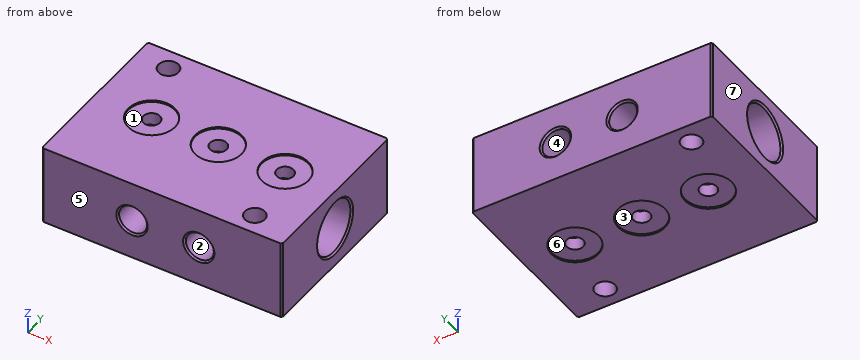
```python
from build123d import *

# Parameters (mm, degrees)
F0_W      = 35
F0_H      = 25
F1_DEPTH  = 12
F2_R      = 4
F3_DEPTH  = 35
F4_R      = 3.5
F4_R_2    = 1.25
F5_DEPTH  = 0.25
F4_R_3    = 1.5
F6_DEPTH  = 25
F7_R      = 1.25
F8_DEPTH  = 25
F10_R     = 2.1
F10_R_2   = 1.25
F11_DEPTH = 6
F9_R      = 2.1
F9_R_2    = 1.25
F12_DEPTH = 6
F13_DEPTH = 1
F14_SIZE  = 0.25
F15_SIZE  = 0.25


with BuildPart() as f1:
    # F0 (on Top) → F1 (new body)
    with BuildSketch(Plane.XY):
        with Locations((17.5, -12.5)):
            Rectangle(F0_W, F0_H)
    extrude(amount=F1_DEPTH)

    # F2 (on face) → F3 (cut, through all)
    with BuildSketch(Plane(origin=(0, 0, 0), x_dir=(0, -1, 0), z_dir=(-1, 0, 0))):
        with Locations((12.5, 6)):
            Circle(F2_R)
    extrude(amount=-F3_DEPTH, mode=Mode.SUBTRACT)

    # F4 (on face) → F6 (cut)
    with BuildSketch(Plane.XY.offset(12)):
        with Locations((30, -22)):
            Circle(F4_R_3)
        with Locations((28.5, -12.5)):
            Circle(F4_R_2)
        with Locations((18.5, -12.5)):
            Circle(F4_R_2)
        with Locations((5, -3)):
            Circle(F4_R_3)
        with Locations((8.5, -12.5)):
            Circle(F4_R_2)
    extrude(amount=-F6_DEPTH, mode=Mode.SUBTRACT)

    # F7 (on face) → F8 (cut)
    with BuildSketch(Plane(origin=(0, 0, 0), x_dir=(-1, 0, 0), z_dir=(0, 1, 0))):
        with Locations((-23.5, 6)):
            Circle(F7_R)
        with Locations((-13.5, 6)):
            Circle(F7_R)
    extrude(amount=-F8_DEPTH, mode=Mode.SUBTRACT)

    # F10 (on face) → F11 (cut)
    with BuildSketch(Plane(origin=(0, 0, 0), x_dir=(-1, 0, 0), z_dir=(0, 1, 0))):
        with Locations((-13.5, 6)):
            Circle(F10_R)
        with Locations((-13.5, 6)):
            Circle(F10_R_2, mode=Mode.SUBTRACT)
        with Locations((-23.5, 6)):
            Circle(F10_R)
        with Locations((-23.5, 6)):
            Circle(F10_R_2, mode=Mode.SUBTRACT)
    extrude(amount=-F11_DEPTH, mode=Mode.SUBTRACT)

    # F9 (on face) → F12 (cut)
    with BuildSketch(Plane.XZ.offset(25)):
        with Locations((13.5, 6)):
            Circle(F9_R)
        with Locations((13.5, 6)):
            Circle(F9_R_2, mode=Mode.SUBTRACT)
        with Locations((23.5, 6)):
            Circle(F9_R)
        with Locations((23.5, 6)):
            Circle(F9_R_2, mode=Mode.SUBTRACT)
    extrude(amount=-F12_DEPTH, mode=Mode.SUBTRACT)

    # F13 (add): a face of the model
    f13_faces = [f1.faces().sort_by_distance(p)[0] for p in [
        (35, -24.7226915075, 6),
    ]]
    extrude(f13_faces, amount=F13_DEPTH)

    # F14
    f14_edges = [f1.edges().sort_by_distance(p)[0] for p in [
        (11.4, -25, 6),
        (21.4, -25, 6),
        (15.6, 0, 6),
        (25.6, 0, 6),
        (36, -8.5, 6),
        (0, -8.5, 6),
    ]]
    chamfer(f14_edges, length=F14_SIZE)

    # F15
    f15_edges = [f1.edges().sort_by_distance(p)[0] for p in [
        (36, -25, 6),
        (36, 0, 6),
        (0, 0, 6),
        (0, -25, 6),
    ]]
    chamfer(f15_edges, length=F15_SIZE)


with BuildPart() as f5:
    # F4 (on face) → F5 (new body)
    with BuildSketch(Plane.XY.offset(12)):
        with Locations((8.5, -12.5)):
            Circle(F4_R)
        with Locations((8.5, -12.5)):
            Circle(F4_R_2, mode=Mode.SUBTRACT)
    extrude(amount=-F5_DEPTH)


with BuildPart() as f5b:
    # F4 (on face) → F5, piece 2 (new body)
    with BuildSketch(Plane.XY.offset(12)):
        with Locations((18.5, -12.5)):
            Circle(F4_R)
        with Locations((18.5, -12.5)):
            Circle(F4_R_2, mode=Mode.SUBTRACT)
    extrude(amount=-F5_DEPTH)


with BuildPart() as f5c:
    # F4 (on face) → F5, piece 3 (new body)
    with BuildSketch(Plane.XY.offset(12)):
        with Locations((28.5, -12.5)):
            Circle(F4_R)
        with Locations((28.5, -12.5)):
            Circle(F4_R_2, mode=Mode.SUBTRACT)
    extrude(amount=-F5_DEPTH)


with BuildPart() as f16_1:
    # F16: instance of F5
    add(f5.part.mirror(Plane.XY))


with BuildPart() as f16_2:
    # F16: instance of F5b
    add(f5b.part.mirror(Plane.XY))


with BuildPart() as f16_3:
    # F16: instance of F5c
    add(f5c.part.mirror(Plane.XY))


with BuildPart() as f16_3_1:
    # F17: moved
    add(f16_3.part.moved(Location((0, 0, 12))))


with BuildPart() as f16_2_1:
    # F17: moved
    add(f16_2.part.moved(Location((0, 0, 12))))


with BuildPart() as f16_1_1:
    # F17: moved
    add(f16_1.part.moved(Location((0, 0, 12))))


with BuildPart() as f1_1:
    add(f1.part)

    # F18: cut F5c, F5, F5b, F16_1, F16_2, F16_3
    add(f5c.part, mode=Mode.SUBTRACT)
    add(f5.part, mode=Mode.SUBTRACT)
    add(f5b.part, mode=Mode.SUBTRACT)
    add(f16_1_1.part, mode=Mode.SUBTRACT)
    add(f16_2_1.part, mode=Mode.SUBTRACT)
    add(f16_3_1.part, mode=Mode.SUBTRACT)


solid = f1_1.part
```
Part model, mm, in its own coordinate system. Face numbers are marked on the shaded views. A direction names the side the tool comes from. Coordinates: 2 decimals unless noted, no trailing zeros. Write each loop counter-clockwise with the first axis right and the second up, starting at its lowest first coordinate (ties: lowest second). Pieces come first, ordered by that corner, then holes.
Item 1: Slice it at A-A (y = -3). Write the cut outline in (x, z), and give its area (3 significant figures).
Item 2: Which spindle directions (+Z, -Z, +X, -X, +Y, -Y) get a long thin tool onto all of the face, cutting with end or side? Do the marked faces 1, 2, 3 and 4. Say none if no direction does.
Item 3: Mould opens along X. For the marked faces 5, 6 and 7 say: released by +X, released by -X, zero draft, split by the parting line, or undercut.
Item 4: Slice it at D-D (y = -7.75). Write the cut outline in (x, z).
Item 5: Pin check, flat tips, straight feed: pin 1 (5 mm diameter, centred on x = 13.5, z = 6, fed in from +Y); pin 2 (1.3 mm diameter, centred on x = 13, z = 7, fed in from -Y); pin 3 (6.5 mm diameter, centred on x = 18.5, y = -12.5, fed in from +Z); pin 4 (2 mm diameter, centred on x = 13.5, z = 5.5, fed in from +Y). Stop position of each tip, or through.
Item 6: Slice it at B-B (x = 13.5). Write the cut outline in (y, z).
Item 7: Probe line 1 (X direction, y = -6.55, z = 6); line 2 (X direction, y = -12.5, z = 1.4); line 3 (Y direction, x = 30, z = 1.5). List the from-to ranges inside material, lowest first.
Item 8: Slice it at C-C (z = 10.75). Write the cut outline in (x, y), and give its area (3 significant figures).
Results found:
1. outline: (0, 0) - (3.5, 0) - (3.5, 12) - (0, 12) - close; (6.5, 0) - (36, 0) - (36, 12) - (6.5, 12) - close; hole circle Ø4.2 at (13.5, 6); hole circle Ø4.2 at (23.5, 6)
1. area: 368 mm2
2. face 1: +Z
2. face 2: -Y
2. face 3: -Z
2. face 4: +Y
3. face 5: zero draft
3. face 6: undercut
3. face 7: released by -X
4. outline: (0, 0) - (36, 0) - (36, 12) - (0, 12) - close; hole circle Ø2.5 at (13.5, 6); hole circle Ø2.5 at (23.5, 6)
5. pin 1: stops at y = 0
5. pin 2: stops at y = -19
5. pin 3: stops at z = 11.75
5. pin 4: stops at y = -6
6. outline: (-25, 0) - (0, 0) - (0, 3.65) - (-0.25, 3.9) - (-6, 3.9) - (-6, 4.75) - (-8.7, 4.75) arc R4 cw to (-16.3, 4.75) - (-19, 4.75) - (-19, 3.9) - (-24.75, 3.9) - (-25, 3.65) - close; (-25, 8.35) - (-24.75, 8.1) - (-19, 8.1) - (-19, 7.25) - (-16.3, 7.25) arc R4 cw to (-8.7, 7.25) - (-6, 7.25) - (-6, 8.1) - (-0.25, 8.1) - (0, 8.35) - (0, 12) - (-25, 12) - close
7. line 1: x = 0 to 12.25, 14.75 to 22.25, 24.75 to 36
7. line 2: x = 0 to 7.25, 9.75 to 17.25, 19.75 to 27.25, 29.75 to 36
7. line 3: y = -25 to -23.5, -20.5 to 0
8. outline: (0, -24.75) - (0.25, -25) - (35.75, -25) - (36, -24.75) - (36, -0.25) - (35.75, 0) - (0.25, 0) - (0, -0.25) - close; hole circle Ø3 at (5, -3); hole circle Ø2.5 at (8.5, -12.5); hole circle Ø2.5 at (18.5, -12.5); hole circle Ø2.5 at (28.5, -12.5); hole circle Ø3 at (30, -22)
8. area: 871 mm2
